from build123d import *

# Parameters (mm, degrees)
SKETCH1_W                 = 94.03907037
SKETCH1_H                 = 136.332098139
BOSS_EXTRUDE1_DEPTH       = 1.5
FILLET1_R                 = 5
SKETCH_PATTERN1_START     = -1
SKETCH_PATTERN1_OUTLINE_R = 1.9304
SKETCH_PATTERN1_DEPTH     = 3
SKETCH4_R                 = 6
CUT_EXTRUDE2_DEPTH        = 136.031781017


with BuildPart() as part:
    # Sketch1 → Boss-Extrude1 (new body)
    with BuildSketch(Plane.XY):
        with Locations((0, 58.406045784)):
            Rectangle(SKETCH1_W, SKETCH1_H)
    extrude(amount=BOSS_EXTRUDE1_DEPTH)

    # Fillet1
    fillet1_edges = [part.edges().sort_by_distance(p)[0] for p in [
        (47.019535185, -9.760003286, 0.75),
        (-47.019535185, -9.760003286, 0.75),
        (-47.019535185, 126.572094853, 0.75),
        (47.019535185, 126.572094853, 0.75),
    ]]
    fillet(fillet1_edges, radius=FILLET1_R)

    # Sketch3 → #24 (0.152) Diameter Hole1 (revolve, cut)
    with BuildSketch(Plane(origin=(-43.009767592, 118.552559669, 1.5), x_dir=(0, -1, 0), z_dir=(1, 0, 0))):
        Polygon((0, 0), (0, 13.859901339), (1.9304, 12.7), (1.9304, 0), align=None)
    revolve(axis=Axis((-43.009767592, 118.552559669, 7.85), (0, 0, -1)), mode=Mode.SUBTRACT)

    # Sketch-Pattern1: read off the stored shape, not the designer's step
    # Sketch-Pattern1 outline → Sketch-Pattern1 (cut)
    with BuildSketch(Plane.XY.offset(SKETCH_PATTERN1_START)):
        with Locations((0, -5.750235693)):
            Circle(SKETCH_PATTERN1_OUTLINE_R)
        with Locations((0, 122.562327261)):
            Circle(SKETCH_PATTERN1_OUTLINE_R)
        with Locations((-43.009767592, -1.740468101)):
            Circle(SKETCH_PATTERN1_OUTLINE_R)
        with Locations((-43.009767592, 46.376743007)):
            Circle(SKETCH_PATTERN1_OUTLINE_R)
        with Locations((43.009767592, -1.740468101)):
            Circle(SKETCH_PATTERN1_OUTLINE_R)
        with Locations((43.009767592, 46.376743007)):
            Circle(SKETCH_PATTERN1_OUTLINE_R)
        with Locations((43.009767592, 118.552559669)):
            Circle(SKETCH_PATTERN1_OUTLINE_R)
    extrude(amount=SKETCH_PATTERN1_DEPTH, mode=Mode.SUBTRACT)

    # Sketch4 → Cut-Extrude2 (cut, through all)
    with BuildSketch(Plane.XY.offset(1.5)):
        with Locations((6.000018773, 79.140018508)):
            Circle(SKETCH4_R)
    extrude(amount=-CUT_EXTRUDE2_DEPTH, mode=Mode.SUBTRACT)


solid = part.part
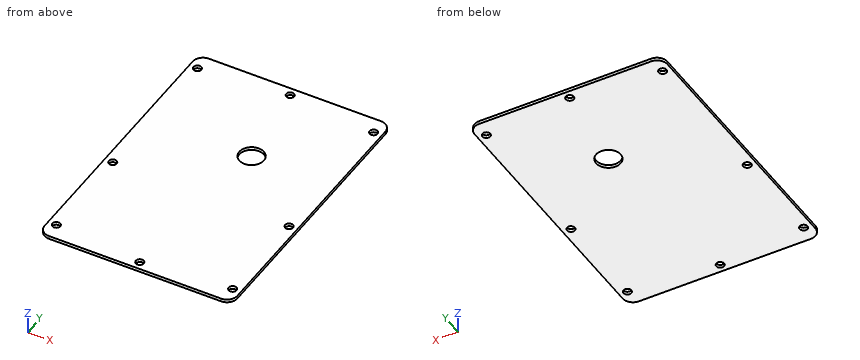
The model under review builds one solid part; all positions refer to its coordinate system, in mm. Give positions to 0.01 mm unless a question says otherwise; leave off trailing zeros. Loops run counter-clockwise (first coordinate to the right, second up) from the corner with the lowest first, then second, coordinate; pieces in that order, holes last. Notation, with made-up numbers: (12, 62) -> (18, 62) arc R34 cw to (18, 96) -> close; hole circle Ø3 at (57.25, -14.75). An arc over 180 degrees is marked (long way). Put each result on its own line as item: value. Start each with the question number.
1. We need section A-A on y = 77. State the section outline as (x, z) points, then the cut area to 3 significant figures.
2. We need section B-B on z = 0.65. State how many separate pieces and enclosed holes the cut face has, then the cut area to 3 significant figures.
3. Wall thickness on probe 1 along X at (y, z) = (46, 1.05); probe 2 along Y at (x, z) = (11, 0.35); probe 3 along Y at (x, z) = (-1.5, 0.1): over which ranges is each line inside the solid? List them lowest first.
Determined:
1. outline: (-47.02, 0) -> (0.39, 0) -> (0.39, 1.5) -> (-47.02, 1.5) -> close; (11.61, 0) -> (47.02, 0) -> (47.02, 1.5) -> (11.61, 1.5) -> close
1. area: 124 mm^2
2. separate pieces: 1
2. enclosed holes: 9
2. area: 12,600 mm^2
3. probe 1: -47.02 to -44.9, -41.12 to 41.12, 44.9 to 47.02
3. probe 2: -9.76 to 75.82, 82.46 to 126.57
3. probe 3: -9.76 to -6.97, -4.54 to 121.35, 123.78 to 126.57
